from build123d import *

# Parameters (mm, degrees)
F0_W     = 10
F0_H     = 8
F1_DEPTH = 5
F2_R     = 4.99999
F3_R     = 1.5
F5_DEPTH = 5
F6_R     = 2.75
F7_DEPTH = 3


# Not quite as in the source:
# - a fillet or chamfer is up to 0.001 mm smaller than in the source, because OpenCascade refuses the exact size


with BuildPart() as f1:
    # F0 (on Top) → F1 (new body)
    with BuildSketch(Plane.XY):
        with Locations((5, 4)):
            Rectangle(F0_W, F0_H)
    extrude(amount=F1_DEPTH)

    # F2 (radius 5 in the source; OpenCascade refuses exactly that, so slightly less here)
    f2_edges = [f1.edges().sort_by_distance(p)[0] for p in [
        (0, 4, 5),
        (10, 4, 5),
    ]]
    fillet(f2_edges, radius=F2_R)

    # F3 (on face) → F5 (cut)
    with BuildSketch(Plane(origin=(0, 0, 0), x_dir=(1, 0, 0), z_dir=(0, 0, -1))):
        with Locations((5, -4)):
            Circle(F3_R)
    extrude(amount=-F5_DEPTH, mode=Mode.SUBTRACT)

    # F6 (on offset) → F7 (cut)
    with BuildSketch(Plane.XY.offset(5)):
        with Locations((5, 4)):
            Circle(F6_R)
    extrude(amount=-F7_DEPTH, mode=Mode.SUBTRACT)


solid = f1.part
Geometry check sheet. Reference: the model listing, model coordinates, mm. A direction names the side the tool comes from. Give positions to 0.01 mm unless a question says otherwise; leave off trailing zeros. Loops run counter-clockwise (first coordinate to the right, second up) from the corner with the lowest first, then second, coordinate; pieces in that order, holes last.
(1) Release check for a two-part mould opening along Y. For faces 1 (the cylindrical face through (5.806, 2.735, 0.986)), 2 (the flat face through (5, 8, 2)), 3 (the flat face through (5, 6, 0)) record: released by +Y, released by -Y, zero draft, split by the parting line, or undercut.
From the geometry:
face 1: undercut
face 2: released by +Y
face 3: zero draft
(2) Depth check by flat-ended pin: pin 1 Ø4.5 at (x, y) = (5, 4) entering from +Z; pin 2 Ø2 at (x, y) = (2.5, 4.5) entering from +Z. Enter the tip coordinate at first touch or a pass-through.
From the geometry:
pin 1: stops at z = 2
pin 2: stops at z = 4.43
(3) Section check C-C on z = 0.9. Record the cut outline in (x, y), then the cut area to 3 significant figures.
From the geometry:
outline: (0.08, 0) - (9.92, 0) - (9.92, 8) - (0.08, 8) - close; hole circle Ø3 at (5, 4)
area: 71.6 mm2
(4) Thickness scan on L1, parallel to Y at x = 5, z = 1.2; L2, parallel to Y at x = 5, z = 4.2; L3, parallel to Z at x = 5.25, y = 6. Record the ranges inside material, lowest first.
From the geometry:
L1: y = 0 to 2.5, 5.5 to 8
L2: y = 0 to 1.25, 6.75 to 8
L3: z = 0 to 2
(5) Section check A-A on x = 3.75. Record the cut outline in (y, z), then the cut area to 3 significant figures.
From the geometry:
outline: (0, 0) - (3.17, 0) - (3.17, 2) - (1.55, 2) - (1.55, 4.84) - (0, 4.84) - close; (4.83, 0) - (8, 0) - (8, 4.84) - (6.45, 4.84) - (6.45, 2) - (4.83, 2) - close
area: 21.5 mm2
(6) Set-up check for faces 4 (the flat face through (6.2, 2.8, 2)), 5 (the cylindrical face through (1, 4, 3)): record each of +Z, -Z, +X, -X, +Y, -Y from which the full face is reachable in a straight line by a thin tool's end or side.
From the geometry:
face 4: +Z
face 5: +Z, -X, +Y, -Y
